Source: CAD feature listing. Evaluate the final solid. Frame: model axes, mm. A direction names the side the tool comes from. Coordinates: 2 decimals unless noted, no trailing zeros. Write each loop counter-clockwise with the first axis right and the second up, starting at its lowest first coordinate (ties: lowest second). Pieces come first, ordered by that corner, then holes. Notation, with made-up numbers: (-1, 28.5) - (42, 28.5) arc R24 ccw to (42, 62.5) - close; hole circle Ø7 at (-28, -11). An arc over 180 degrees is marked (long way). One line per question, with ' | ' between items.
Autodesk Inventor part; units mm, degrees
ref_plane "YZ Plane" through (0, 0, 0) normal (1, 0, 0) x (0, 1, 0)
ref_plane "XZ Plane" through (0, 0, 0) normal (0, 1, 0) x (-1, 0, 0)
ref_plane "XY Plane" through (0, 0, 0) normal (0, 0, 1) x (1, 0, 0)
sketch "Sketch1" plane through (0, 0, 0) normal (0, 1, 0) x (-1, 0, 0)
  line L0 (10.6592, 60.325) -> (-7.8828, 60.325)
  line L1 (-7.8828, 60.325) -> (-7.8828, -12.7)
  line L2 (-7.8828, -12.7) -> (10.6592, -12.7)
  line L3 (10.6592, 54.61) -> (-1.5328, 54.61)
  line L4 (-1.5328, 54.61) -> (-1.5328, 28.575)
  line L5 (-1.5328, 28.575) -> (10.6592, 28.575)
  line L6 (10.6592, 19.05) -> (-1.5328, 19.05)
  line L7 (-1.5328, 19.05) -> (-1.5328, -6.35)
  line L8 (-1.5328, -6.35) -> (10.6592, -6.35)
  line L9 (10.6592, -12.7) -> (10.6592, -6.35)
  line L10 (10.6592, 19.05) -> (10.6592, 28.575)
  line L11 (10.6592, 54.61) -> (10.6592, 60.325)
  point P0 (0, 0)
  dimension "d0" = 18.542
  dimension "d3" = 6.35
  dimension "d4" = 9.525
  dimension "d5" = 5.715
  dimension "d7" = 0
  dimension "d8" = 26.035
  dimension "d9" = 25.4
  dimension "d25" = 0
  dimension "d26" = 0
extrude "Extrusion1" add sketch "Sketch1" along normal blind 101.6
sketch "Sketch2" plane through (1.5328, 0, -6.35) normal (-1, 0, 0) x (0, 0, 1)
  line L0 (0, 0) -> (0, 101.6)
  line L1 (0, 0) -> (25.4, 0)
  point P0 (6.35, 0)
  point P1 (12.7, 25.4)
  point P2 (12.7, 50.8)
  point P3 (12.7, 76.2)
  dimension "d12" = 12.7
  dimension "d13" = 25.4
  dimension "d14" = 25.4
  dimension "d15" = 0
  dimension "d16" = 0
  dimension "d17" = 25.4
hole "Hole1" at (1.5328, 25.4, 6.35) at (1.5328, 50.8, 6.35) at (1.5328, 76.2, 6.35) direction (1, 0, 0) diameter 4.826 depth 25.4 tip angle 118
sketch "Sketch3" plane through (0, 101.6, 0) normal (0, 1, 0) x (1, 0, 0)
  line L0 (1.5328, -28.575) -> (-10.7917, -28.1446)
  line L1 (-10.7917, -28.1446) -> (-10.7917, -28.575)
  line L2 (-10.6592, -28.575) -> (1.5328, -28.575)
  line L3 (-10.7917, -28.575) -> (1.5328, -28.575)
  point P0 (0, 0)
  dimension "d27" = 2
extrude "Extrusion2" cut sketch "Sketch3" against normal blind 111.125
sketch "Sketch4" plane through (0, 101.6, 0) normal (0, 1, 0) x (1, 0, 0)
  line L0 (1.5328, -54.61) -> (-12.9577, -54.61)
  line L1 (-12.9577, -54.61) -> (-12.9577, -55.116)
  line L2 (-12.9577, -55.116) -> (1.5328, -54.61)
  point P0 (0, 0)
  dimension "d30" = 2
extrude "Extrusion3" cut sketch "Sketch4" against normal blind 119.0625
sketch "Sketch5" plane through (0, 101.6, 0) normal (0, 1, 0) x (1, 0, 0)
  line L0 (-10.6592, -60.325) -> (7.8828, -60.325)
  line L1 (7.8828, -60.325) -> (-13.0423, -59.5943)
  line L2 (-13.0423, -59.5943) -> (-13.0009, -60.325)
  line L3 (-13.0009, -60.325) -> (7.8828, -60.325)
  point P0 (0, 0)
  dimension "d33" = 2
extrude "Extrusion4" cut sketch "Sketch5" against normal blind 196.85
sketch "Sketch6" plane through (0, 101.6, 0) normal (0, 1, 0) x (1, 0, 0)
  line L0 (7.8828, 12.7) -> (-10.6592, 12.7)
  line L1 (7.8828, 12.7) -> (-16.8119, 12.7)
  line L2 (-16.8119, 12.7) -> (-16.8119, 11.8376)
  line L3 (7.8828, -60.325) -> (7.8828, 12.7)
  line L4 (-16.8119, 11.8376) -> (7.8828, 12.7)
  point P0 (0, 0)
  dimension "d36" = 2
extrude "Extrusion5" cut sketch "Sketch6" against normal blind 334.9625
sketch "Sketch8" plane through (1.5328, 0, -6.35) normal (-1, 0, 0) x (0, 0, 1)
  line L0 (0, 0) -> (25.4, 0)
  circle A0 centre (12.7, 25.4) radius 2.413
  circle A1 centre (12.7, 50.8) radius 2.413
  circle A2 centre (12.7, 76.2) radius 2.413
  line L1 (25.4, 0) -> (25.4, 101.6)
  line L2 (0, 0) -> (25.4, 0)
  line L3 (25.4, 0) -> (25.4, 101.6)
  line L4 (25.4, 101.6) -> (0, 101.6)
  line L5 (0, 101.6) -> (0, 0)
  circle A3 centre (12.7, 25.4) radius 2.413
  circle A4 centre (12.7, 50.8) radius 2.413
  circle A5 centre (12.7, 76.2) radius 2.413
  point P0 (6.35, 0)
extrude "Extrusion7" add sketch "Sketch8" along normal blind 0.7937
sketch "Sketch13" plane through (1.5328, 0, 28.575) normal (-1, 0, 0) x (0, 0, 1)
  line L0 (19.995, 46.69) -> (9.7479, 40.7738)
  line L1 (9.7479, 40.7738) -> (9.7479, 52.6062)
  line L2 (9.7479, 52.6062) -> (19.995, 46.69)
  point P0 (-28.575, 0)
  point P1 (13.1636, 46.69)
extrude "Extrusion10" cut sketch "Sketch13" against normal blind 241.3
sketch "Sketch14" plane through (1.5328, 0, 28.575) normal (-1, 0, 0) x (0, 0, 1)
  circle A0 centre (14.1651, 19.3247) radius 4.4158
  point P0 (-28.575, 0)
extrude "Extrusion11" cut sketch "Sketch14" against normal blind 58.7375
sketch "Sketch15" plane through (-10.6592, 0, 19.05) normal (-1, 0, 0) x (0, 0, 1)
  line L0 (-42.6377, -21.5043) -> (50.0762, -21.5043)
  line L1 (50.0762, -21.5043) -> (50.0762, 3.175)
  line L2 (50.0762, 3.175) -> (-42.6377, 3.175)
  line L3 (-42.6377, 3.175) -> (-42.6377, -21.5043)
  line L4 (-43.9771, 109.6049) -> (47.6951, 109.6049)
  line L5 (47.6951, 109.6049) -> (47.6951, 98.425)
  line L6 (47.6951, 98.425) -> (-43.9771, 98.425)
  line L7 (-43.9771, 98.425) -> (-43.9771, 109.6049)
  line L8 (0, 101.6) -> (9.0992, 101.6)
  line L9 (0, 0) -> (9.0992, 0)
  point P0 (-19.05, 0)
  dimension "d55" = 3.175
  dimension "d56" = 3.175
extrude "Extrusion12" cut sketch "Sketch15" against normal blind 58.7375
equation "\"d0\" = ElvDelWidth"
equation "\"d3\" = ElvDelFrontTabLength"
equation "\"d9\" = ElvBeamWidth"
equation "\"d10\" = ElvDelHeight"
equation "\"ElvBeamWidth\" = 25.4"
equation "\"ElvDelWidth\" = 18.542"
equation "\"ElvDelHeight\" = 101.6"
equation "\"ElvDelFrontTabLength\" = 6.35"
equation "\"ElvDelDepth\" = 6.35"
equation "\"d2\" = ElvDelDepth"
equation "\"ElvCrossBeamLength\" = 304.8"
equation "\"ElvFixedBeamLength\" = 990.6"
equation "\"ElvMiddleBeamLength\" = 990.6"
equation "\"ElvFrontBeamLength\" = 990.6"
equation "\"ElvEndEffectLength\" = 431.8"
equation "\"ElvWallWidth\" = 1.5875"
equation "\"ElvTopBeamLength\" = 457.2"
equation "\"ElvHoleFromFront\" = 25.4"
equation "\"ElvHoleFromMid\" = 38.1"
equation "\"ElvHoleFromFixed\" = 50.8"
equation "\"ElvHoleFromBottom\" = 38.1"
equation "\"ElvRivetPlateLength\" = 76.2"
equation "\"ElvDelMiddleTabLength\" = 6.35"
properties part number "ElvDelV5" material "Acetal Resin, White"
Item 1: Cut plane D-D on y = 50.8. Return loops of the section in (x, z) (3 decimals), and give its area (3 significant figures).
Check sheet entries:
outline: (-10.659, -12.052) - (7.883, -12.7) - (7.883, 3.937) - (0.739, 3.937) - (0.739, -6.35) - (-10.659, -6.35) - close; (-10.659, 19.05) - (0.739, 19.05) - (0.739, 8.763) - (7.883, 8.763) - (7.883, 38.323) - (1.533, 38.323) - (1.533, 28.575) - (-10.659, 28.149) - close; (-10.659, 55.036) - (1.533, 54.61) - (1.533, 41.451) - (7.883, 41.451) - (7.883, 60.325) - (-10.659, 59.678) - close | area: 676 mm²
Item 2: Cut plane A-A on z = 6.35. Return loops of the section in (x, y) (3 decimals), and give its area (3 significant figures).
Check sheet entries:
outline: (0.739, 3.175) - (7.883, 3.175) - (7.883, 22.987) - (0.739, 22.987) - close; (0.739, 27.813) - (7.883, 27.813) - (7.883, 48.387) - (0.739, 48.387) - close; (0.739, 53.213) - (7.883, 53.213) - (7.883, 73.787) - (0.739, 73.787) - close; (0.739, 78.613) - (7.883, 78.613) - (7.883, 98.425) - (0.739, 98.425) - close | area: 577 mm²
Item 3: Mould query, pull axis Y, two halves, no side actions, for faces 1 (the face through (1, 3.175, 24)), 2 (the face through (5, 47, 38.323)), 3 (the face through (0.739, 51, 3)), 4 (the face through (4.663, 22.309, 39.485)). Classes: pulls with the +Y half, pulls with the -Y half, needs draft (parallel to the pull), parting line crosses it, or undercut.
Check sheet entries:
face 1: pulls with the -Y half | face 2: undercut | face 3: needs draft | face 4: undercut
Item 4: Access query for faces 5 (the face through (-10.659, 50, -9)), 6 (the face through (1.533, 50, 45)), 7 (the face through (4.66, 49.69, 43.37)). Directions: +Z, -Z, +X, -X, +Y, -Y. A direction counts if a zero-diameter tool reaches every point of the face in a straight line with its end or side. Return the directions, or none.
Check sheet entries:
face 5: +Z, -Z, -X, +Y, -Y | face 6: -X, +Y, -Y | face 7: +X, -X
Item 5: Pin query (flat end, axial travel): pin 1 Ø3.5 at (x, y) = (-7, 48) entering from +Z; pin 2 Ø10 at (y, z) = (21.5, 3.5) entering from -X; pin 3 Ø1.9 at (x, y) = (3.5, 48) entering from +Z. Return the tip coordinate at first contact, or that it passes through.
Check sheet entries:
pin 1: z = 59.87 | pin 2: x = 0.74 | pin 3: z = 60.21
Item 6: Cut plane C-C on x = -4.5. Return loops of the section in (y, z) (3 decimals), and give its area (3 significant figures).
Check sheet entries:
outline: (3.175, -12.268) - (98.425, -12.268) - (98.425, -6.35) - (3.175, -6.35) - close; (3.175, 19.05) - (98.425, 19.05) - (98.425, 28.364) - (3.175, 28.364) - close; (3.175, 54.821) - (98.425, 54.821) - (98.425, 59.893) - (3.175, 59.893) - close | area: 1,930 mm²
Item 7: Ray query, line 1 along Y through (x, z) = (4.5, 6.35) (3 decimals); line 2 along Z through (x, y) = (-7.5, 20); line 3 along Z through (x, y) = (-8, 94). Return the intervals inside material, ascending. Write a range as [from, to].
Check sheet entries:
line 1: [3.175, 22.987], [27.813, 48.387], [53.213, 73.787], [78.613, 98.425] | line 2: [-12.16, -6.35], [19.05, 28.26], [54.93, 59.79] | line 3: [-12.15, -6.35], [19.05, 28.24], [54.94, 59.77]
Item 8: Cut plane B-B on y = 25.4. Return loops of the section in (x, z) (3 decimals).
Check sheet entries:
outline: (-10.659, -12.052) - (7.883, -12.7) - (7.883, 3.937) - (0.739, 3.937) - (0.739, -6.35) - (-10.659, -6.35) - close; (-10.659, 19.05) - (0.739, 19.05) - (0.739, 8.763) - (7.883, 8.763) - (7.883, 60.325) - (-10.659, 59.678) - (-10.659, 55.036) - (1.533, 54.61) - (1.533, 28.575) - (-10.659, 28.149) - close
